The model under review builds one solid part; all positions refer to its coordinate system, in mm. A direction names the side the tool comes from. Give positions to 0.01 mm unless a question says otherwise; leave off trailing zeros. Order: outer loops, then holes, each group sorted by start corner. A loop starts at its lowest first (then second) coordinate and runs counter-clockwise, first axis right, second up. Notation, with made-up numbers: (-29.5, -28.75) - (11.5, -28.75) arc R20 ccw to (11.5, -21.75) - close; hole circle Ø10 at (0.5, 57.5). An arc over 180 degrees is marked (long way). Answer as CSV lines item,"result". Start each with the question number.
Autodesk Inventor part; units mm, degrees
ref_plane "YZ Plane" through (0, 0, 0) normal (1, 0, 0) x (0, 1, 0)
ref_plane "XZ Plane" through (0, 0, 0) normal (0, 1, 0) x (-1, 0, 0)
ref_plane "XY Plane" through (0, 0, 0) normal (0, 0, 1) x (1, 0, 0)
sketch "Sketch1" plane through (0, 0, 0) normal (0, 0, 1) x (1, 0, 0)
  line L0 (0, 0) -> (100, 0) construction
  line L1 (0, -5.1674) -> (100, -5.1674)
  line L2 (100, 5.1674) -> (0, 5.1674)
  arc A0 (0, 5.1674) -> (0, -5.1674) centre (0, 0) ccw
  arc A1 (100, -5.1674) -> (100, 5.1674) centre (100, 0) ccw
  point P0 (50, 0)
  dimension "d0" = 100
extrude "Extrusion1" add sketch "Sketch1" along normal blind 3
sketch "Sketch2" plane through (0, 0, 3) normal (0, 0, 1) x (1, 0, 0)
  circle A0 centre (0, 0) radius 2.125
  dimension "d3" = 4.25
extrude "Extrusion2" add sketch "Sketch2" along normal blind 3 and the other way blind 6
sketch "Sketch3" plane through (0, 0, 3) normal (0, 0, 1) x (1, 0, 0)
  circle A0 centre (140.404, 0) radius 2.125
  point P0 (0, 0)
  dimension "d8" = 4.25
extrude "Extrusion3" cut sketch "Sketch3" against normal blind 3
sketch "Sketch4" plane through (0, 0, 3) normal (0, 0, 1) x (1, 0, 0)
  circle A0 centre (120.4729, 0) radius 2.125
  point P0 (0, 0)
  dimension "d11" = 4.25
extrude "Extrusion4" cut sketch "Sketch4" against normal blind 10
sketch "Sketch5" plane through (0, 0, 3) normal (0, 0, 1) x (1, 0, 0)
  circle A0 centre (98.4795, 0) radius 2.125
  point P0 (0, 0)
  dimension "d14" = 4.25
extrude "Extrusion5" cut sketch "Sketch5" against normal blind 10
properties part number "connector linkage"
Item 1: Take a section at C-C on x = 92. Write out the cut boundary in (y, z).
Item 2: Clearance check with flat-ended pins moving along their axes: pin 1 (1.5 mm diameter, centred on y = -1.5, z = 0, fed in from +X); pin 2 (3 mm diameter, centred on x = 81.5, y = -1.5, fed in from -Z); pin 3 (2 mm diameter, centred on y = 1, z = 3.5, fed in from -X). State where each tip first meets the part, or that it passes through.
Item 3: For line 1 along Z through (x, y) = (23.5, 0.5); line 2 along Y through (x, z) = (0.5, 4.5), list the stretches that pass through material, from the lowest coordinate up.
Item 4: Take a section at D-D on y = -4.25. Write out the cut boundary in (x, z).
Item 5: Mouldability with a two-part tool opening along X and no side actions: class faces 3 (the face through (49, -5.167, 1)), 4 (the face through (1.142, -1.792, 4.479)), 5 (the face through (100.506, 0.638, 1.521)), 6 (the face through (-5.166, -0.114, 1.479)) as released by +X, released by -X, zero draft, split by the parting line, or undercut.
Item 6: Take a section at A-A on y = 0. Write out the cut boundary in (x, z) (1 decimal).
Item 7: Machinability: for faces 1 (the face through (1.142, 1.792, -1.479)), 2 (the face through (0, 0, -3)), which of the approach directions +Z, -Z, +X, -X, +Y, -Y give a long, thin tool a straight path to every point of the face, cutting with its end or side? Answer none if there is none.
Data:
1,outline,"(-5.17, 0) - (5.17, 0) - (5.17, 3) - (-5.17, 3) - close"
2,pin 1,"stops at x = 105.11"
2,pin 2,"stops at z = 0"
2,pin 3,"stops at x = -5.17"
3,line 1,"z = 0 to 3"
3,line 2,"y = -2.07 to 2.07"
4,outline,"(-2.94, 0) - (102.94, 0) - (102.94, 3) - (-2.94, 3) - close"
5,face 3,"zero draft"
5,face 4,"split by the parting line"
5,face 5,"undercut"
5,face 6,"released by -X"
6,outline,"(-5.2, 0) - (-2.1, 0) - (-2.1, -3) - (2.1, -3) - (2.1, 0) - (96.4, 0) - (96.4, 3) - (2.1, 3) - (2.1, 6) - (-2.1, 6) - (-2.1, 3) - (-5.2, 3) - close; (100.6, 0) - (105.2, 0) - (105.2, 3) - (100.6, 3) - close"
7,face 1,"-Z"
7,face 2,"-Z, +X, -X, +Y, -Y"
